For this review, take the finished solid that the model builds, in its own axes (mm). A direction names the side the tool comes from. Coordinates: 2 decimals unless noted, no trailing zeros. Put each result on its own line as item: value. Start each with the question number.
Item 1: The part is to be moulded in two halves that separate along Z. For faces 1 (the conical face through (35.78, -13.24, 24.68)), 2 (the flat face through (-1, -25, -39.51)), 3 (the flat face through (-1, 0, 1)), 4 (the conical face through (-34.97, -13.24, 24.68)), say which applies: +Z half, -Z half, draft (parallel to the pull), parting line (faces both ways), or undercut.
Item 2: To check wall thickness, follow L1, parallel to Z at x = -35.5, y = -7. State the ranges of the line that lie inside material, in increasing order.
Item 3: Insertion check: P1, Ø6.5, axis at x = -35.38, z = -24.51, coming from the +Y side; P2, Ø4, axis at x = 35.38, z = 24.51, coming from the +Y side. Each pin has a flat end and moves straight along its axis. Give the tip position at first contact, or say it passes through.
Item 4: For faces 5 (the cylindrical face through (-32.878, -7.612, -24.62)), 6 (the flat face through (50.375, -25, -1)), list the 3-axis set-ups (+Z, -Z, +X, -X, +Y, -Y) from which the entire face can be reached by the end or side of a thin tool; tool diameter is ignored.
```python
from build123d import *

# Parameters (mm, degrees)
F0_W           = 100.7501929998
F0_H           = 79.0197588503
F1_DEPTH       = 50
F2_D           = 5
F2_DEPTH       = 12
F2_CSINK_D     = 11.2
F2_CSINK_ANGLE = 90
F2_TIP         = 1.5021515476


with BuildPart() as f1:
    # F0 (on Front) → F1 (new body)
    with BuildSketch(Plane.XZ):
        Rectangle(F0_W, F0_H)
    extrude(amount=F1_DEPTH)

    # F2
    with Locations(Plane(origin=(0, 0, 0), x_dir=(1, 0, 0), z_dir=(0, 1, 0))):
        with Locations((-35.3750964999, -24.5098794252), (35.3750964999, -24.5098794252), (35.3750964999, 24.5098794252), (-35.3750964999, 24.5098794252)):
            CounterSinkHole(F2_D / 2, F2_CSINK_D / 2, depth=F2_DEPTH, counter_sink_angle=F2_CSINK_ANGLE)
            with Locations((0, 0, -(F2_DEPTH + F2_TIP / 2))):  # 118° drill point
                Cone(0, F2_D / 2, F2_TIP, mode=Mode.SUBTRACT)


solid = f1.part
```
Return value:
1. face 1: undercut
1. face 2: -Z half
1. face 3: draft
1. face 4: undercut
2. L1: -39.51 to -27.01, -22.01 to 22.01, 27.01 to 39.51
3. P1: y = -2.35
3. P2: y = -12.3
4. face 5: +Y
4. face 6: +Z, -Z, +X, +Y, -Y
